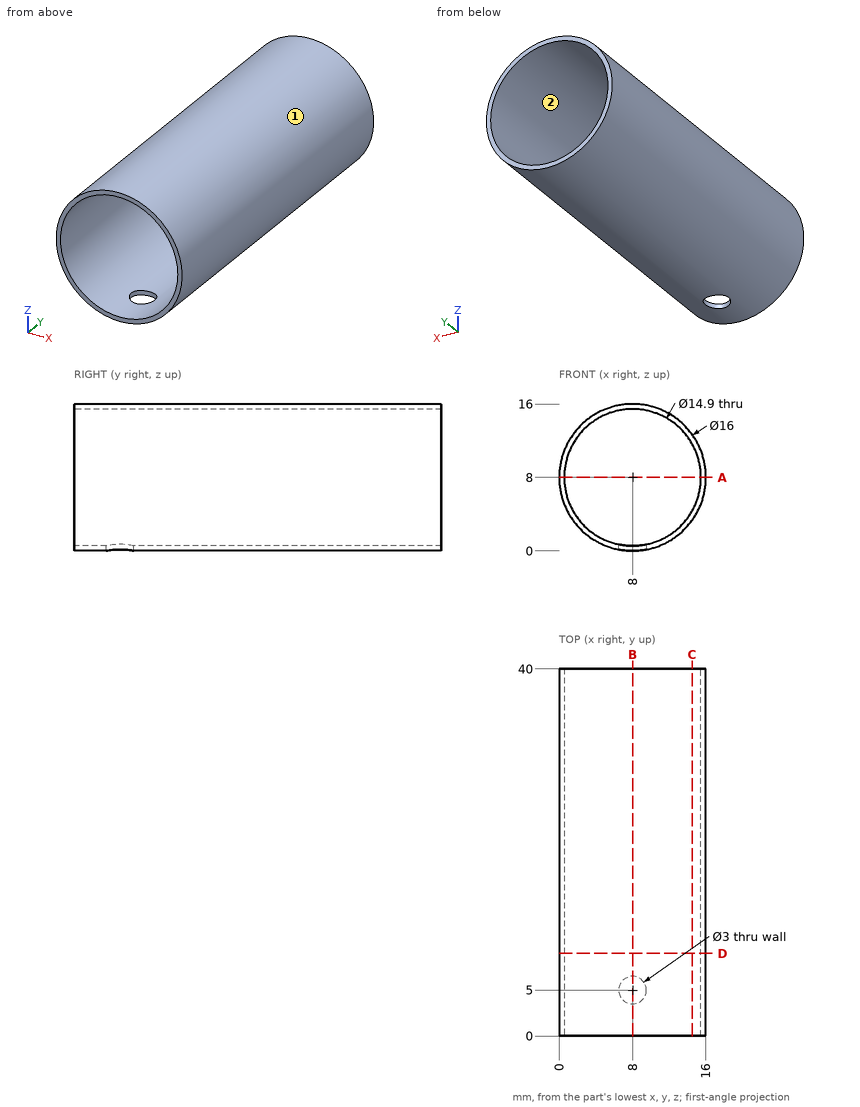
Verification items for this drawing (mm, ordinates from the low corner). Coordinates: 2 decimals unless noted, no trailing zeros. Write each loop counter-clockwise with the first axis right and the second up, starting at its lowest first coordinate (ties: lowest second). Pieces come first, ordered by that corner, then holes. Notation, with made-up numbers: M 72.25,31.5 L 109.25,31.5 A33 cw 109.25,64.5 Z; hole C -12.5,-7 d2. An arc over 180 degrees is marked long. One line per item, written item: value. Start each with the question number.
(1) Depth check by flat-ended pin: pin 1 (1.5 mm diameter, centred on x = 6.5, y = 31, fed in from -Z); pin 2 (1.5 mm diameter, centred on y = 13, z = 10.5, fed in from +X). Enter the tip coordinate at first touch or a pass-through.
(2) Release check for a two-part mould opening along X. For the marked faces 1 and 2 record: released by +X, released by -X, zero draft, split by the parting line, or undercut.
(3) Sectioned sample at A-A, the plane z = 8. Enter the section's corners in (x, y).
(4) Sectioned sample at B-B, the plane x = 8. Enter the section's corners in (y, z), and give its area (4 significant figures).
(5) Sectioned sample at D-D, the plane y = 9. Enter the section's corners in (x, z), and give its area (3 significant figures).
(6) Scan lines: line 1 along X through (y, z) = (8.5, 8.25); line 2 along Y through (x, z) = (8, 0.2); line 3 along Z through (x, y) = (4.75, 19). Record each from-to range of solid material in increasing order. Write a range as [from, to].
(7) Sectioned sample at C-C, the plane x = 14.5. Enter the section's corners in (y, z), and give its area (3 significant figures).
Filled sheet:
1. pin 1: z = 0.04
1. pin 2: x = 15.81
2. face 1: split by the parting line
2. face 2: undercut
3. outline: M 0,0 L 0.55,0 L 0.55,40 L 0,40 Z; M 15.45,0 L 16,0 L 16,40 L 15.45,40 Z
4. outline: M 0,0 L 3.5,0 L 3.5,0.55 L 0,0.55 Z; M 0,15.45 L 40,15.45 L 40,16 L 0,16 Z; M 6.5,0 L 40,0 L 40,0.55 L 6.5,0.55 Z
4. area: 42.35 mm²
5. outline: C 8,8 d16; hole C 8,8 d14.9
5. area: 26.7 mm²
6. line 1: [0, 0.55], [15.45, 16]
6. line 2: [0, 3.5], [6.5, 40]
6. line 3: [0.69, 1.3], [14.7, 15.31]
7. outline: M 0,3.34 L 40,3.34 L 40,4.36 L 0,4.36 Z; M 0,11.64 L 40,11.64 L 40,12.66 L 0,12.66 Z
7. area: 81.9 mm²
